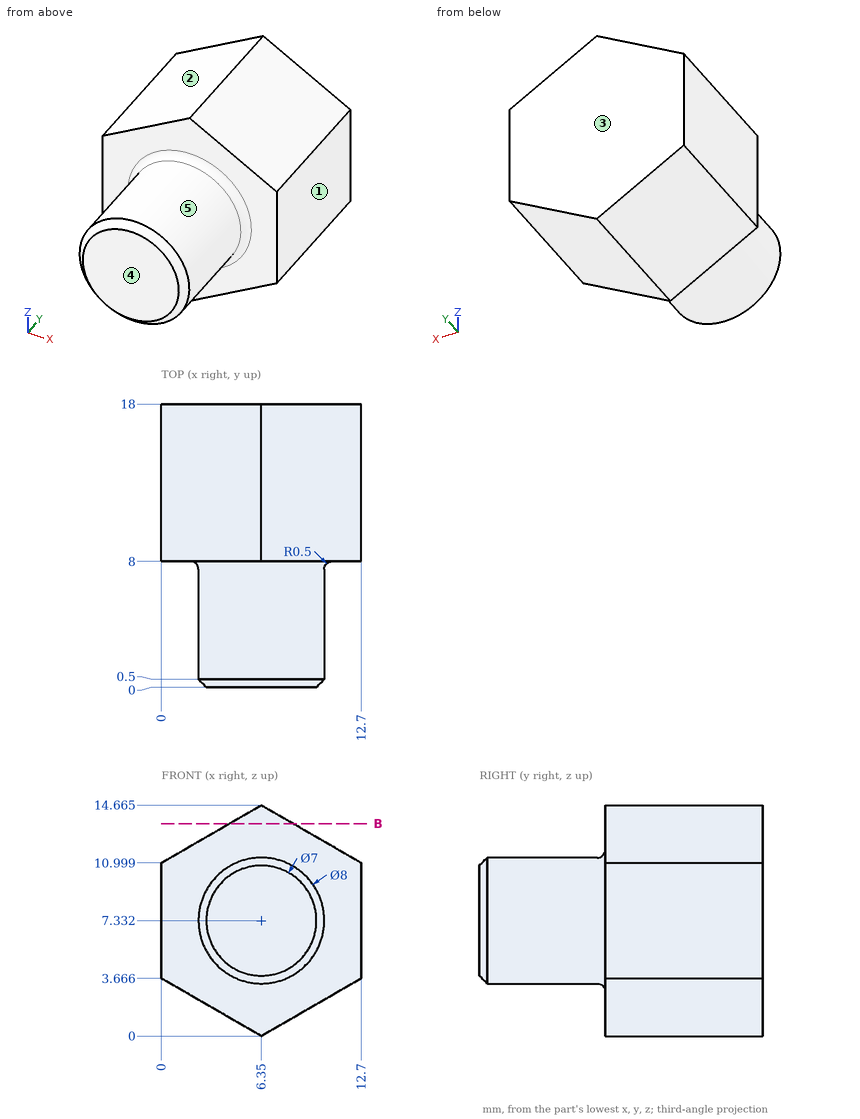
Source: three-view drawing plus pictorial views. Frame: mm from the lowest corner of the part. A direction names the side the tool comes from. Coordinates: 2 decimals unless noted, no trailing zeros. Order: outer loops, then holes, each group sorted by start corner. A loop starts at its lowest first (then second) coordinate and runs counter-clockwise, first axis right, second up.
Item 1: Material intervals for line 1 (Y direction, x = 2, z = 5.5); line 2 (Z direction, x = 6.5, y = 7.5) (1 decimal); line 3 (Z direction, x = 8, y = 15.5), sorted ascending.
Output values:
line 1: y = 8 to 18
line 2: z = 3.3 to 11.3
line 3: z = 0.95 to 13.71
Item 2: Set-up query: the marked faces 4 and 5. Return all of +Z, -Z, +X, -X, +Y, -Y with unobstructed straight access to the full face (end or side cutting, diameter ignored); none if empty.
Output values:
face 4: +Z, -Z, +X, -X, -Y
face 5: -Y
Item 3: Cut plane B-B (z = 13.5). Return loops of the section in (x, y).
Output values:
outline: (4.33, 8) - (8.37, 8) - (8.37, 18) - (4.33, 18) - close
Item 4: First-contact query: P1, Ø2, axis at y = 4.5, z = 6.5, coming from the -X side; P2, Ø4, axis at x = 3.5, y = 7.5, coming from the -Z side; P3, Ø2, axis at x = 10.5, y = 3.5, coming from the -Z side (1 decimal). Flat tips, straight axial feed; report the tip coordinate or a pass-through.
Output values:
P1: stops at x = 2.35
P2: stops at z = 0.53
P3: stops at z = 4.9
Item 5: Pull-direction query (X, two-part tool) for the marked faces 1, 2 and 3; classes: pulls with the +X half, pulls with the -X half, needs draft (parallel to the pull), parting line crosses it, or undercut.
Output values:
face 1: pulls with the +X half
face 2: pulls with the -X half
face 3: needs draft
